Here's how the part is built. I have some questions about the finished solid (model axes, mm). Round coordinates to 2 decimals unless told otherwise and drop trailing zeros. Order: outer loops, then holes, each group sorted by start corner. A loop starts at its lowest first (then second) coordinate and runs counter-clockwise, first axis right, second up. Notation, with made-up numbers: (87, -13.5) -> (129, -13.5) arc R10 ccw to (129, 3.5) -> close; hole circle Ø4 at (-34, 14). An arc over 180 degrees is marked (long way). Use a Markdown table: item, result. Add a question column.
(1) I want a section at B-B, the plane x = -4.5. Please give me the cut outline in (y, z).
(2) I'm going to push flat-ended pins straight in: P1, Ø6, axis at x = 4, y = 3.5, coming from the +Z side; P2, Ø4, axis at x = 1, z = 3.5, coming from the +Y side; P3, Ø4, axis at y = 3.5, z = 3, coming from the -X side. Where does each tip first touch, or does it pass through?
(3) If I drill on probe 1 along Z at (x, y) = (1, 6); probe 2 along Z at (x, y) = (-0.25, 5.25); probe 3 along X at (y, z) = (-5.5, -6.25), over which ranges is the centre line in solid material (lowest first)?
(4) I want a section at A-A, the plane z = 5.25. Please give me the cut outline in (x, y), then the cut area to 3 significant figures.
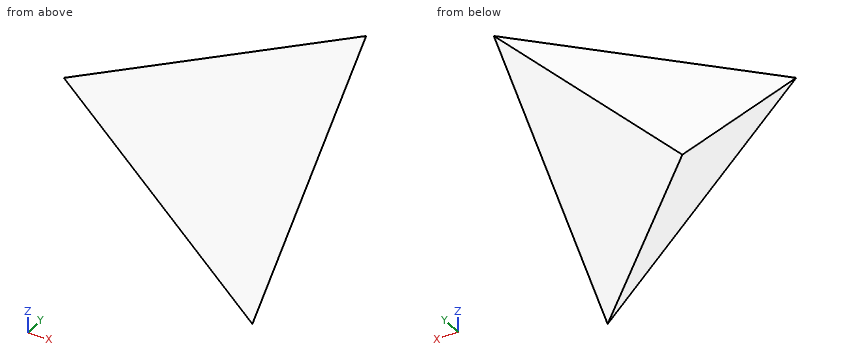
from build123d import *

# Parameters (mm, degrees)
CIRPATTERN2_2_ANGLE   = 180
CIRPATTERN2_2_5_ANGLE = 180


with BuildPart() as body_1:
    # Sketch12 → Surface-Plane4: a flat surface bounded by the sketch
    with BuildSketch(Plane(origin=(-2.357022604, -2.357022604, -2.357022604), x_dir=(0.4082482904638632, 0.4082482904638626, -0.8164965809277261), z_dir=(0.5773502691896264, 0.5773502691896254, 0.5773502691896256)), mode=Mode.PRIVATE) as surface_plane4_1_region:
        Polygon((-11.547005384, 0), (5.773502692, -10), (5.773502692, 10), align=None)
    surface_plane4_1 = surface_plane4_1_region.sketch.faces()[0]
    # CirPattern2: a copy of that surface (a pattern of surface bodies)
    cirpattern2_2 = surface_plane4_1.rotate(Axis((0, 0, 0), (0, 1, 0)), CIRPATTERN2_2_ANGLE)
    # Sketch11 → Surface-Plane3: a flat surface bounded by the sketch
    with BuildSketch(Plane(origin=(2.357022604, 2.357022604, -2.357022604), x_dir=(0.40824829046386335, 0.4082482904638629, 0.8164965809277259), z_dir=(-0.577350269189626, -0.5773502691896255, 0.577350269189626)), mode=Mode.PRIVATE) as surface_plane3_3_region:
        Polygon((-5.773502692, -10), (11.547005384, 0), (-5.773502692, 10), align=None)
    surface_plane3_3 = surface_plane3_3_region.sketch.faces()[0]
    # Sketch11 → Surface-Plane3: a flat surface bounded by the sketch
    with BuildSketch(Plane(origin=(2.357022604, 2.357022604, -2.357022604), x_dir=(0.40824829046386335, 0.4082482904638629, 0.8164965809277259), z_dir=(-0.577350269189626, -0.5773502691896255, 0.577350269189626)), mode=Mode.PRIVATE) as surface_plane3_4_region:
        Polygon((-5.773502692, -10), (11.547005384, 0), (-5.773502692, 10), align=None)
    surface_plane3_4 = surface_plane3_4_region.sketch.faces()[0]
    # CirPattern2 2: a copy of that surface (a pattern of surface bodies)
    cirpattern2_2_5 = surface_plane3_4.rotate(Axis((0, 0, 0), (0, 1, 0)), CIRPATTERN2_2_5_ANGLE)
    # Sketch12 → Surface-Plane4: a flat surface bounded by the sketch
    with BuildSketch(Plane(origin=(-2.357022604, -2.357022604, -2.357022604), x_dir=(0.4082482904638632, 0.4082482904638626, -0.8164965809277261), z_dir=(0.5773502691896264, 0.5773502691896254, 0.5773502691896256)), mode=Mode.PRIVATE) as surface_plane4_6_region:
        Polygon((-11.547005384, 0), (5.773502692, -10), (5.773502692, 10), align=None)
    surface_plane4_6 = surface_plane4_6_region.sketch.faces()[0]
    # Surface-Knit2: the surfaces knitted into a closed skin and filled: a solid
    add(Solid(Shell(Face.sew_faces(cirpattern2_2.faces() + surface_plane3_3.faces() + cirpattern2_2_5.faces() + surface_plane4_6.faces())[0])))


solid = body_1.part
Taken from the geometry:
| question | item | result |
|---|---|---|
| 1 | outline | (-7.07, 4.5) -> (4.5, -7.07) -> (7.07, -4.5) -> (-4.5, 7.07) -> close |
| 2 | P1 | stops at z = 7.07 |
| 2 | P2 | stops at y = 7.07 |
| 2 | P3 | stops at x = -3.4 |
| 3 | probe 1 | z = -0.07 to 2.07 |
| 3 | probe 2 | z = -2.07 to 1.57 |
| 3 | probe 3 | x = 4.68 to 6.32 |
| 4 | outline | (-7.07, -5.25) -> (-5.25, -7.07) -> (7.07, 5.25) -> (5.25, 7.07) -> close |
| 4 | area | 44.9 mm2 |
